Part model, mm, in its own coordinate system. A direction names the side the tool comes from. Coordinates: 2 decimals unless noted, no trailing zeros. Order: outer loops, then holes, each group sorted by start corner. A loop starts at its lowest first (then second) coordinate and runs counter-clockwise, first axis right, second up.
```python
from build123d import *

# Parameters (mm, degrees)
SKETCH1_W           = 65
SKETCH1_H           = 65
BOSS_EXTRUDE1_DEPTH = 5
BOSS_EXTRUDE3_DEPTH = 7.5
BOSS_EXTRUDE5_DEPTH = 85.7
SKETCH8_R           = 2.55
CUT_EXTRUDE4_DEPTH  = 102.615648401
SKETCH8_3_R         = 4.1
SKETCH8_3_R_2       = 2.55
CUT_EXTRUDE5_DEPTH  = 3.75
SKETCH9_R           = 2.55
BOSS_EXTRUDE6_DEPTH = 7.5
SKETCH10_R          = 4.1
CUT_EXTRUDE6_DEPTH  = 3.75
BOSS_EXTRUDE7_DEPTH = 32.5
CUT_EXTRUDE7_DEPTH  = 32.5
FILLET1_R           = 5
SKETCH14_W          = 91.4
SKETCH14_H          = 5
CUT_EXTRUDE8_DEPTH  = 10
FILLET2_R           = 1.5
FILLET7_R           = 2
BOSS_EXTRUDE9_DEPTH = 65
FILLET9_R           = 2


with BuildPart() as part:
    # Sketch1 → Boss-Extrude1 (new body)
    with BuildSketch(Plane.XY):
        Rectangle(SKETCH1_W, SKETCH1_H)
    extrude(amount=BOSS_EXTRUDE1_DEPTH)



with BuildPart() as body_2:
    # Sketch4 → Boss-Extrude3 (new body)
    with BuildSketch(Plane.ZY.offset(53.2)):
        Polygon((5, -12.5), (-15, -32.5), (-15, -52.5), (5, -32.5), align=None)
    extrude(amount=-BOSS_EXTRUDE3_DEPTH)


with BuildPart() as part_1:
    add(part.part)

    add(body_2.part)  # Boss-Extrude5 merges body 2
    # Sketch7 → Boss-Extrude5 (add)
    with BuildSketch(Plane(origin=(-53.2, 0, 0), x_dir=(0, 0, -1), z_dir=(1, 0, 0))):
        Polygon((-5, -32.5), (0, -32.5), (0, -17.5), (-5, -12.5), align=None)
    boss_extrude5 = extrude(amount=BOSS_EXTRUDE5_DEPTH)

    # Sketch8 → Cut-Extrude4 (cut, through all)
    with BuildSketch(Plane.ZY.offset(53.2)):
        with Locations((-7.5, -35)):
            Circle(SKETCH8_R)
    extrude(amount=-CUT_EXTRUDE4_DEPTH, mode=Mode.SUBTRACT)

    # Sketch8<3> → Cut-Extrude5 (cut)
    with BuildSketch(Plane.ZY.offset(53.2)):
        with Locations((-7.5, -35)):
            Circle(SKETCH8_3_R)
        with Locations((-7.5, -35)):
            Circle(SKETCH8_3_R_2, mode=Mode.SUBTRACT)
    extrude(amount=-CUT_EXTRUDE5_DEPTH, mode=Mode.SUBTRACT)

    # Mirror5: Boss-Extrude5 across plane
    add(boss_extrude5.mirror(Plane(origin=(0, 0, 0), x_dir=(0, 0, 1), z_dir=(1, 0, 0))))

    # Sketch9 → Boss-Extrude6 (add)
    with BuildSketch(Plane(origin=(53.2, 0, 0), x_dir=(0, 0, -1), z_dir=(1, 0, 0))):
        Polygon((0, -17.5), (-5, -12.5), (-5, -32.5), (15, -52.5), (15, -32.5), align=None)
        with Locations(Location((7.5, -35, 0), (0, 0, 180))):
            Circle(SKETCH9_R, mode=Mode.SUBTRACT)
    extrude(amount=-BOSS_EXTRUDE6_DEPTH)

    # Sketch10 → Cut-Extrude6 (cut)
    with BuildSketch(Plane(origin=(53.2, 0, 0), x_dir=(0, 0, -1), z_dir=(1, 0, 0))):
        with Locations(Location((7.5, -35, 0), (0, 0, 180))):
            Circle(SKETCH10_R)
    extrude(amount=-CUT_EXTRUDE6_DEPTH, mode=Mode.SUBTRACT)

    # Sketch11 → Boss-Extrude7 (add, symmetric)
    with BuildSketch(Plane(origin=(0, 0, 0), x_dir=(0, 0, -1), z_dir=(1, 0, 0))):
        with BuildLine():
            Line((-5, -12.5), (-5, -32.5))
            Line((-5, -32.5), (0, -32.5))
            Line((0, -32.5), (0, -17.5))
            ThreePointArc((0, -17.5), (1.245268577, -11.245121626), (3.482006161, -5.272584286))
            ThreePointArc((3.482006161, -5.272584286), (5.362849311, 0.228699546), (6, 6.007603745))
            Line((6, 6.007603745), (6, 32.5))
            Line((6, 32.5), (1, 32.5))
            Line((1, 32.5), (1, 4.967162469))
            ThreePointArc((1, 4.967162469), (0.129503325, 0.320168795), (-1.970810175, -3.915512716))
            ThreePointArc((-1.970810175, -3.915512716), (-4.043682345, -8.010758246), (-5, -12.5))
        make_face()
    extrude(amount=BOSS_EXTRUDE7_DEPTH, both=True)

    # Sketch13 → Cut-Extrude7 (cut, symmetric)
    with BuildSketch(Plane(origin=(0, 0, 0), x_dir=(0, 0, -1), z_dir=(1, 0, 0))):
        with BuildLine():
            ThreePointArc((-1.970810175, -3.915512716), (-4.043682345, -8.010758246), (-5, -12.5))
            Line((-5, -12.5), (-5, 32.5))
            Line((-5, 32.5), (1, 32.5))
            Line((1, 32.5), (1, 4.967162469))
            ThreePointArc((1, 4.967162469), (0.129503325, 0.320168795), (-1.970810175, -3.915512716))
        make_face()
    extrude(amount=CUT_EXTRUDE7_DEPTH, both=True, mode=Mode.SUBTRACT)

    # Fillet1
    fillet1_edges = [part_1.edges().sort_by_distance(p)[0] for p in [
        (-49.45, -32.5, -15),
        (-49.45, -52.5, -15),
        (49.45, -32.5, -15),
        (49.45, -52.5, -15),
    ]]
    fillet(fillet1_edges, radius=FILLET1_R)

    # Sketch14 → Cut-Extrude8 (cut)
    with BuildSketch(Plane.XY.offset(5)):
        with Locations((0, -30)):
            Rectangle(SKETCH14_W, SKETCH14_H)
    extrude(amount=-CUT_EXTRUDE8_DEPTH, mode=Mode.SUBTRACT)

    # Fillet2
    fillet2_edges = [part_1.edges().sort_by_distance(p)[0] for p in [
        (0, -27.5, 0),
        (49.45, -32.5, 5),
        (-49.45, -32.5, 5),
    ]]
    fillet(fillet2_edges, radius=FILLET2_R)

    # Fillet7
    fillet7_edges = [part_1.edges().sort_by_distance(p)[0] for p in [
        (32.5, 32.5, -3.5),
        (-32.5, 32.5, -3.5),
    ]]
    fillet(fillet7_edges, radius=FILLET7_R)

    # Sketch16 → Boss-Extrude9 (add)
    with BuildSketch(Plane.ZY.offset(32.5)):
        with BuildLine():
            Line((-6, 6.007603745), (-6, -7.821383753))
            ThreePointArc((-6, -7.821383753), (-4.378318661, -13.515143769), (0, -17.5))
            Line((0, -17.5), (2.89677664, -14.60322336))
            Line((2.89677664, -14.60322336), (-3.112770549, 6.007603745))
            Line((-3.112770549, 6.007603745), (-6, 6.007603745))
        make_face()
    extrude(amount=-BOSS_EXTRUDE9_DEPTH)

    # Fillet9
    fillet9_edges = [part_1.edges().sort_by_distance(p)[0] for p in [
        (32.5, 11.339308123, -6),
        (-32.5, 11.339308123, -6),
        (0, 32.5, -6),
        (31.914213562, 31.914213562, -6),
        (-31.914213562, 31.914213562, -6),
        (-32.5, -13.515143769, -4.378318661),
        (32.5, -13.515143769, -4.378318661),
    ]]
    fillet(fillet9_edges, radius=FILLET9_R)


solid = part_1.part
```
(1) Slice it at C-C, the plane x = -2.5. Give the cut face in (y, z).
(2) Slice it at A-A, the plane x = -35.5. Give the cut face in (y, z).
(3) Pull direction X, two halves, no side cores. Call faces 4 (the face through (45.7, -34.37, -4.86)), 5 (the face through (1, -20, 5)), 6 (the face through (-49.45, -38, -8)): +X half, -X half, draft (parallel to the pull), parting line (faces both ways), or undercut.
(4) Slice it at B-B, the plane y = -20. Give the cut face in (x, z), then the cut area to 4 significant figures.
(5) Probe line 1 (X direction, y = -41.5, z = -6.5); line 2 (Z direction, x = 30.5, y = 16); line 3 (Z direction, x = 48, y = -35). List the from-to ranges inside material, lowest first.
(6) Tool access for faces 1 (the face through (1, -22, 0)), 2 (the face through (50, -38, -15)), 3 (the face through (49.45, -32, -8)): list every direction of +Z, -Z, +X, -X, +Y, -Y with a clear straight run to the whole face (end or side of a thin tool).
(7) Drop flat-ended pins along their axis: pin 1 (10 mm diameter, centred on y = 18.5, z = 0.5, fed in from +X); pin 2 (4 mm diameter, centred on x = 10, y = -23, fed in from -Z); pin 3 (3 mm diameter, centred on y = 2, z = -3, fed in from -X). Give the stop position or say it passes through.
Here are the results:
1. outline: (-27.5, 1.5) arc R1.5 ccw to (-26, 0) - (-17.5, 0) arc R10.81 ccw to (-7.82, -6) - (30.5, -6) arc R2 ccw to (32.5, -4) - (32.5, -1) - (4.97, -1) arc R17.24 cw to (-3.92, 1.97) arc R17.79 ccw to (-12.5, 5) - (-27.5, 5) - close
2. outline: (-27.5, 1.5) arc R1.5 ccw to (-26, 0) - (-17.5, 0) - (-12.5, 5) - (-27.5, 5) - close
3. face 4: undercut
3. face 5: draft
3. face 6: -X half
4. outline: (-53.2, -2.5) - (-45.7, -2.5) - (-45.7, 0) - (45.7, 0) - (45.7, -2.5) - (53.2, -2.5) - (53.2, 5) - (-53.2, 5) - close
4. area: 569.5 mm2
5. line 1: x = -53.2 to -45.7, 45.7 to 53.2
5. line 2: z = -6 to -1
5. line 3: z = -15 to -10.05, -4.95 to 2.5
6. face 1: -Z, -Y
6. face 2: -Z, +X, -X, +Y, -Y
6. face 3: +X
7. pin 1: stops at x = 32.5
7. pin 2: stops at z = 0
7. pin 3: stops at x = -32.5
